Here's how the part is built. I have some questions about the finished solid (model axes, mm). Coordinates: 2 decimals unless noted, no trailing zeros. Write each loop counter-clockwise with the first axis right and the second up, starting at its lowest first coordinate (ties: lowest second). Pieces come first, ordered by that corner, then holes. Notation, with made-up numbers: (65, -34.75) -> (122, -34.75) arc R30 cw to (122, -0.75) -> close; hole circle Ø5 at (56, 55). An arc over 180 degrees is marked (long way). Use a Markdown table: item, result. Add a question column.
Item 1: If I drill on line 1 along Y through (x, z) = (1.35, 32); line 2 along Y through (x, z) = (1.05, 28.5); line 3 along Z through (x, y) = (0.7, 39), over which ranges is the centre line in solid material (lowest first)? Write a range as from..to.
Item 2: Imagine slicing it at D-D, the plane x = 0.7. Write out the boundary of the cut face in (y, z), and give its area (3 significant figures).
Item 3: Imagine slicing it at B-B, the plane y = 44.5. Write out the boundary of the cut face in (x, z).
Item 4: Imagine slicing it at A-A, the plane z = 26. Write out the boundary of the cut face in (x, y).
Item 5: Imagine slicing it at C-C, the plane z = 35. Write out the boundary of the cut face in (x, y).
```python
from build123d import *

# Parameters (mm, degrees)
SKETCH_1_W          = 95
SKETCH_1_H          = 38.85
EXTRUDE_1_DEPTH     = 1
SKETCH_2_W          = 10.1
SKETCH_2_H          = 28.4
SKETCH_2_W_2        = 23.6
SKETCH_2_H_2        = 25.25
CUT_EXTRUDE_1_DEPTH = 10


with BuildPart() as part:
    # Эскиз1 → Бобышка-Вытянуть1 (new body)
    with BuildSketch(Plane(origin=(0.5, 0, 0), x_dir=(0, -1, 0), z_dir=(-1, 0, 0))):
        with Locations((-53.35, 22.825)):
            Rectangle(SKETCH_1_W, SKETCH_1_H)
    extrude(amount=-EXTRUDE_1_DEPTH)

    # Эскиз2 → Вырез-Вытянуть1 (cut)
    with BuildSketch(Plane.ZY.offset(-0.5)):
        with Locations((35.85, 40.15)):
            Rectangle(SKETCH_2_W, SKETCH_2_H)
        with Locations((29.1, 81.275)):
            Rectangle(SKETCH_2_W_2, SKETCH_2_H_2)
    extrude(amount=-CUT_EXTRUDE_1_DEPTH, mode=Mode.SUBTRACT)


solid = part.part
```
Ans:
| question | item | result |
|---|---|---|
| 1 | line 1 | y = 5.85..25.95, 54.35..68.65, 93.9..100.85 |
| 1 | line 2 | y = 5.85..68.65, 93.9..100.85 |
| 1 | line 3 | z = 3.4..30.8, 40.9..42.25 |
| 2 | outline | (5.85, 3.4) -> (100.85, 3.4) -> (100.85, 42.25) -> (5.85, 42.25) -> close; hole (25.95, 30.8) -> (54.35, 30.8) -> (54.35, 40.9) -> (25.95, 40.9) -> close; hole (68.65, 17.3) -> (93.9, 17.3) -> (93.9, 40.9) -> (68.65, 40.9) -> close |
| 2 | area | 2,810 mm^2 |
| 3 | outline | (0.5, 3.4) -> (1.5, 3.4) -> (1.5, 30.8) -> (0.5, 30.8) -> close; (0.5, 40.9) -> (1.5, 40.9) -> (1.5, 42.25) -> (0.5, 42.25) -> close |
| 4 | outline | (0.5, 5.85) -> (1.5, 5.85) -> (1.5, 68.65) -> (0.5, 68.65) -> close; (0.5, 93.9) -> (1.5, 93.9) -> (1.5, 100.85) -> (0.5, 100.85) -> close |
| 5 | outline | (0.5, 5.85) -> (1.5, 5.85) -> (1.5, 25.95) -> (0.5, 25.95) -> close; (0.5, 54.35) -> (1.5, 54.35) -> (1.5, 68.65) -> (0.5, 68.65) -> close; (0.5, 93.9) -> (1.5, 93.9) -> (1.5, 100.85) -> (0.5, 100.85) -> close |
